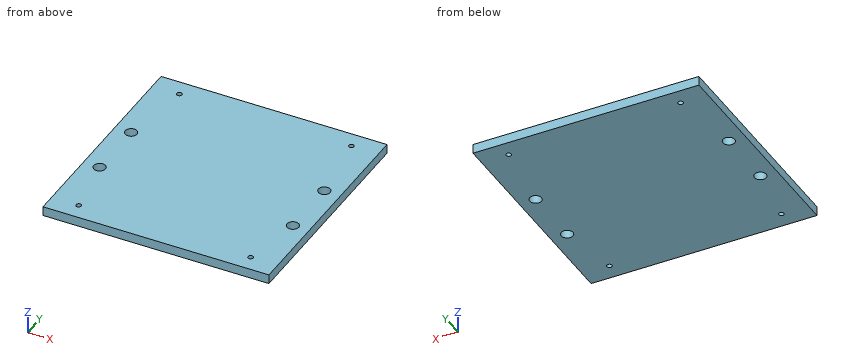
```python
from build123d import *

# Parameters (mm, degrees)
SKETCH1_W                          = 152.4
SKETCH1_H                          = 152.4
BOSS_EXTRUDE1_DEPTH                = 6.35
F_5_16_0_3125_DIAMETER_HOLE1_D     = 7.9375
F_5_16_0_3125_DIAMETER_HOLE1_DEPTH = 6.35
F_8_32_TAPPED_HOLE1_D              = 3.4544
F_8_32_TAPPED_HOLE1_DEPTH          = 6.35


with BuildPart() as part:
    # Sketch1 → Boss-Extrude1 (new body)
    with BuildSketch(Plane.XY):
        with Locations((0, 113)):
            Rectangle(SKETCH1_W, SKETCH1_H)
    extrude(amount=BOSS_EXTRUDE1_DEPTH)

    # 5/16 (0.3125) Diameter Hole1
    with Locations(Plane(origin=(0, 0, 0), x_dir=(-1, 0, 0), z_dir=(0, 0, -1))):
        with Locations((65.1764, 88.807), (65.1764, 129.447), (-65.1764, 129.447), (-65.1764, 88.807)):
            Hole(F_5_16_0_3125_DIAMETER_HOLE1_D / 2, depth=F_5_16_0_3125_DIAMETER_HOLE1_DEPTH)

    # #8-32 Tapped Hole1
    with Locations(Plane(origin=(0, 0, 0), x_dir=(-1, 0, 0), z_dir=(0, 0, -1))):
        with Locations((-58, 178), (58, 178), (58, 48), (-58, 48)):
            Hole(F_8_32_TAPPED_HOLE1_D / 2, depth=F_8_32_TAPPED_HOLE1_DEPTH)


solid = part.part
```
The listing builds one solid part. Answer for the finished solid, in the listing's coordinates (mm). Round coordinates to 2 decimals unless told otherwise and drop trailing zeros. Write each loop counter-clockwise with the first axis right and the second up, starting at its lowest first coordinate (ties: lowest second). Pieces come first, ordered by that corner, then holes. Notation, with made-up numbers: (40.5, 27.25) -> (79.5, 27.25) arc R26 cw to (79.5, 42.25) -> close; hole circle Ø6 at (64, 73.5). An arc over 180 degrees is marked (long way). Answer as a JSON object with one key per item and string values. Group by question number.
Q1. Straight lines are drawn through the part: line 1 along X through (y, z) = (178, 4.5); line 2 along Y through (x, z) = (-58, 4); line 3 along Y through (x, z) = (-59.5, 6). For each, find the intervals that lie inside material, in ascending order.
Q2. Section B-B (x = -58) is taken. Write down the section's boundary in (y, z).
Q3. Section A-A (y = 48) is taken. Write down the section's boundary in (x, z).
Check values:
{
 "1": {"line 1": "-76.2 to -59.73, -56.27 to 56.27, 59.73 to 76.2", "line 2": "36.8 to 46.27, 49.73 to 176.27, 179.73 to 189.2", "line 3": "36.8 to 47.14, 48.86 to 177.14, 178.86 to 189.2"},
 "2": {"outline": "(36.8, 0) -> (46.27, 0) -> (46.27, 6.35) -> (36.8, 6.35) -> close; (49.73, 0) -> (176.27, 0) -> (176.27, 6.35) -> (49.73, 6.35) -> close; (179.73, 0) -> (189.2, 0) -> (189.2, 6.35) -> (179.73, 6.35) -> close"},
 "3": {"outline": "(-76.2, 0) -> (-59.73, 0) -> (-59.73, 6.35) -> (-76.2, 6.35) -> close; (-56.27, 0) -> (56.27, 0) -> (56.27, 6.35) -> (-56.27, 6.35) -> close; (59.73, 0) -> (76.2, 0) -> (76.2, 6.35) -> (59.73, 6.35) -> close"}
}
